Read the model definition and answer for the solid it produces. Units are mm, in the model's axes. A direction names the side the tool comes from. Give positions to 0.01 mm unless a question says otherwise; leave off trailing zeros. Order: outer loops, then holes, each group sorted by start corner. A loop starts at its lowest first (then second) coordinate and runs counter-clockwise, first axis right, second up. Notation, with made-up numbers: (-37, 56.5) - (-15, 56.5) arc R23 cw to (-15, 91.5) - close; hole circle Ø6 at (-2.75, -28.75). An arc over 180 degrees is marked (long way). Write item = value, one per line.
```python
from build123d import *

# Parameters (mm, degrees)
SKETCH2_W               = 4
SKETCH2_H               = 20.325154634
CUT_EXTRUDE1_DEPTH      = 16
CUT_EXTRUDE1_DEPTH_BACK = 16


with BuildPart() as part:
    # Sketch1 → Revolve1 (revolve)
    with BuildSketch(Plane.XY):
        with BuildLine():
            Line((0, 53), (0, 0))
            Line((0, 0), (10.15, 0))
            Line((10.15, 0), (10.15, 38))
            Line((10.15, 38), (15, 38))
            ThreePointArc((15, 38), (10.606601718, 48.606601718), (0, 53))
        make_face()
    revolve(axis=Axis((0, 53, 0), (0, -1, 0)))

    # Sketch2 → Cut-Extrude1 (cut, two sides)
    with BuildSketch(Plane.XY) as cut_extrude1_sk:
        with Locations((0, 51.162577317)):
            Rectangle(SKETCH2_W, SKETCH2_H)
    extrude(amount=CUT_EXTRUDE1_DEPTH, mode=Mode.SUBTRACT)
    extrude(cut_extrude1_sk.sketch, amount=-CUT_EXTRUDE1_DEPTH_BACK, mode=Mode.SUBTRACT)


solid = part.part
```
1. Section A-A (z = 0) is taken. Determine the outline of the cut face in (x, y), and give its area (3 significant figures).
Recorded:
outline = (-15, 38) - (-10.15, 38) - (-10.15, 0) - (10.15, 0) - (10.15, 38) - (15, 38) arc R15 ccw to (2, 52.87) - (2, 41) - (-2, 41) - (-2, 52.87) arc R15 ccw to start
area = 1,080 mm^2
2. Straight lines are drawn through the part: L1, parallel to X at y = 49, z = 3; L2, parallel to Z at x = -2.5, y = 39.5; L3, parallel to Y at x = 3.25, z = 5.75. For each, find the intervals that lie inside material, in ascending order. Write a range as [from, to].
Recorded:
L1 = [-9.75, -2], [2, 9.75]
L2 = [-14.71, 14.71]
L3 = [0, 51.47]
3. Determine the mould class of faces 1 (the face through (-3, 38, -10)), 2 (the face through (-2, 46, 0)), 3 (the face through (0, 41, 0)), 4 (the face through (-8.05, 19.27, -6.18)) for opening direction X: +X half, -X half, draft (parallel to the pull), parting line (faces both ways), or undercut.
Recorded:
face_1 = draft
face_2 = undercut
face_3 = undercut
face_4 = parting line
4. For faces 5 (the face through (0, 0, 0)), 6 (the face through (2, 46, 0)), determine the directions among +Z, -Z, +X, -X, +Y, -Y from which every point of the face is accessible in a straight line to the end or side of a thin tool.
Recorded:
face_5 = +Z, -Z, +X, -X, -Y
face_6 = +Z, -Z, +Y
5. Flat-ended cylindrical pins translate along their axes: pin 1 (9.5 mm diameter, centred on y = 49, z = 4, fed in from -X); pin 2 (4 mm diameter, centred on x = 2, y = 18, fed in from -Z); pin 3 (3 mm diameter, centred on x = 9, y = 32.5, fed in from +Z). Find the tip coordinate at first contact, or state that the pin passes through.
Recorded:
pin_1 = -13.29
pin_2 = -10.15
pin_3 = 6.84
6. Section C-C (y = 22.5) is taken. Determine the outline of the cut face in (x, z), and give its area (3 significant figures).
Recorded:
outline = circle Ø20.3 at (0, 0)
area = 324 mm^2
7. Section D-D (x = 6) is taken. Determine the outline of the cut face in (y, z), and give its area (3 significant figures).
Recorded:
outline = (0, -8.19) - (38, -8.19) - (38, -13.75) arc R13.75 ccw to (38, 13.75) - (38, 8.19) - (0, 8.19) - close
area = 919 mm^2
8. Section B-B (x = 0) is taken. Determine the outline of the cut face in (y, z), and give its area (3 significant figures).
Recorded:
outline = (0, -10.15) - (38, -10.15) - (38, -15) arc R15 ccw to (41, -14.7) - (41, 14.7) arc R15 ccw to (38, 15) - (38, 10.15) - (0, 10.15) - close
area = 861 mm^2
